The figure shows three views and two pictorial views of one solid part (mm, origin at its lowest corner). Answer the questions. A direction names the side the tool comes from. Round coordinates to 2 decimals unless told otherwise and drop trailing zeros. Order: outer loops, then holes, each group sorted by start corner. A loop starts at its lowest first (then second) coordinate and runs counter-clockwise, first axis right, second up. Notation, with made-up numbers: (-11.75, 80) - (38.25, 80) arc R20 ccw to (38.25, 90) - close; hole circle Ø9 at (73.5, 31.5). An arc over 180 degrees is marked (long way). Answer as a JSON object with one key per item and string values. Group by question number.
Q1. Given pin 1 Ø1.5 at (x, z) = (1.5, 12.5) entering from +Y; pin 2 Ø1.2 at (x, z) = (1.5, 18.5) entering from -Y; pin 3 Ø1.2 at (x, y) = (1.5, 1) entering from +Z, each flat-ended and moving along its own axis, determine where each tip first touches the part or whether it passes through.
Q2. Consider line 1 (Y direction, x = 2.2, z = 17.25); line 2 (Z direction, x = 2.9, y = 1.75); line 3 (Z direction, x = 0.3, y = 11.25). Determine where each line is inside the solid, lowest interval first.
Q3. A tool of negligible diameter and unlimited length cuts with its end or side. For the marked faces 4, 5 and 6, from which of +Z, -Z, +X, -X, +Y, -Y can it reach the whole face along a straight path? Write none if from no direction.
Q4. A cutting plane is placed at B-B on x = 1.15. Determine the outline of the cut face in (y, z).
Q5. A cutting plane is placed at C-C on y = 18.5. Determine the outline of the cut face in (x, z).
Q6. A cutting plane is placed at D-D on z = 4. Determine the outline of the cut face in (x, y).
Q7. The mould has two halves that part along Z. Classify the marked faces 1, 2 and 3: pulls with the +Z half, pulls with the -Z half, needs draft (parallel to the pull), parting line crosses it, or undercut.
Q8. A cutting plane is placed at A-A on z = 18.5. Determine the outline of the cut face in (x, y).
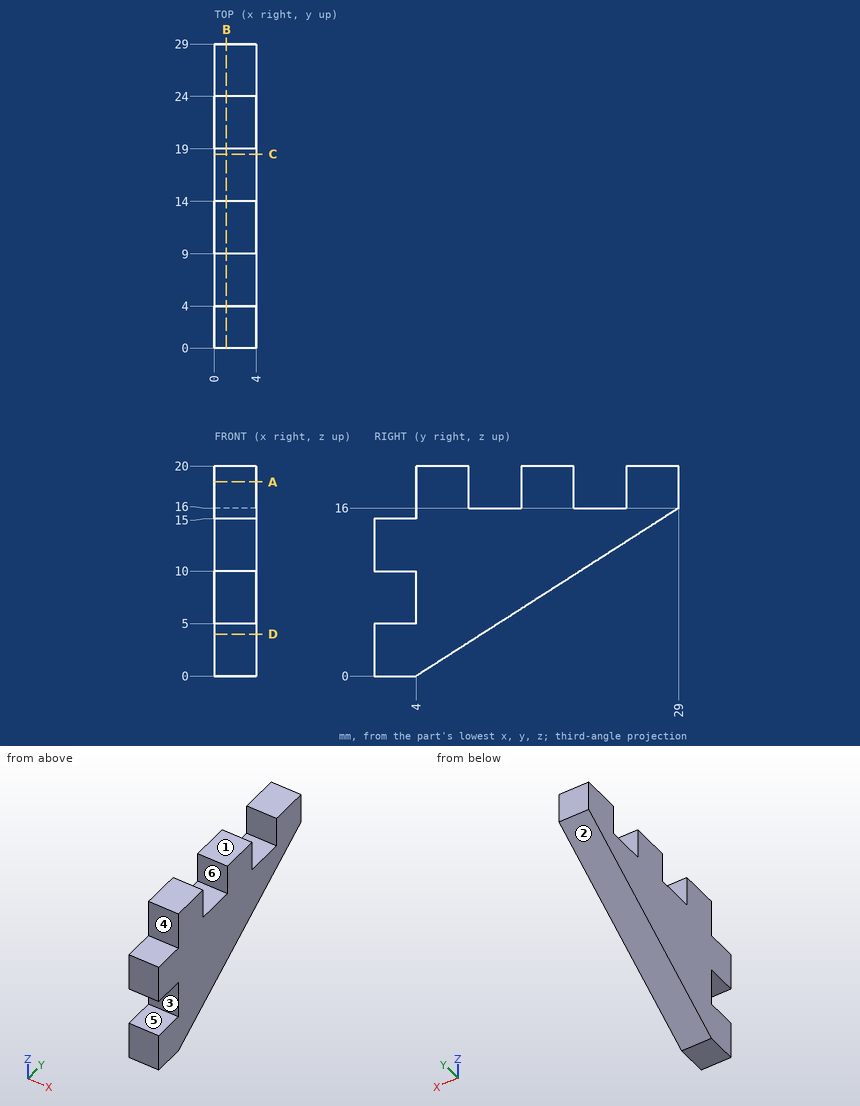
Result set:
{
 "1": {"pin 1": "stops at y = 24.7", "pin 2": "stops at y = 4", "pin 3": "stops at z = 15"},
 "2": {"line 1": "y = 4 to 9, 14 to 19, 24 to 29", "line 2": "z = 0 to 5, 10 to 15", "line 3": "z = 4.64 to 16"},
 "3": {"face 4": "+Z, +X, -X, -Y", "face 5": "+X, -X, -Y", "face 6": "+Z, +X, -X"},
 "4": {"outline": "(0, 0) - (4, 0) - (29, 16) - (29, 20) - (24, 20) - (24, 16) - (19, 16) - (19, 20) - (14, 20) - (14, 16) - (9, 16) - (9, 20) - (4, 20) - (4, 15) - (0, 15) - (0, 10) - (4, 10) - (4, 5) - (0, 5) - close"},
 "5": {"outline": "(0, 9.28) - (4, 9.28) - (4, 20) - (0, 20) - close"},
 "6": {"outline": "(0, 0) - (4, 0) - (4, 10.25) - (0, 10.25) - close"},
 "7": {"face 1": "pulls with the +Z half", "face 2": "pulls with the -Z half", "face 3": "undercut"},
 "8": {"outline": "(0, 4) - (4, 4) - (4, 9) - (0, 9) - close; (0, 14) - (4, 14) - (4, 19) - (0, 19) - close; (0, 24) - (4, 24) - (4, 29) - (0, 29) - close"}
}
